Model file for the job. Use its own axes, mm. A direction names the side the tool comes from. Round coordinates to 2 decimals unless told otherwise and drop trailing zeros. Loops run counter-clockwise (first coordinate to the right, second up) from the corner with the lowest first, then second, coordinate; pieces in that order, holes last. Notation, with made-up numbers: (6.5, -4) - (36.5, -4) arc R24 ccw to (36.5, 30) - close; hole circle Ø3 at (-31.5, -13.75). An arc over 180 degrees is marked (long way). Use one line per item in the form item = value.
from build123d import *

# Parameters (mm, degrees)
ESQUISSE1_W                   = 270
ESQUISSE1_H                   = 213
BOSS_EXTRU_1_DEPTH            = 6
ESQUISSE3_R                   = 9.475
ESQUISSE3_R_2                 = 1.5
ENL_V_MAT_EXTRU_1_DEPTH       = 10
ENL_V_MAT_EXTRU_11_DEPTH      = 173.055950202
ENL_V_MAT_EXTRU_11_DEPTH_BACK = 173.055950202
ESQUISSE6_W                   = 40
ESQUISSE6_H                   = 6
BOSS_EXTRU_2_DEPTH            = 6
ESQUISSE7_W                   = 6
ESQUISSE7_H                   = 30
ESQUISSE7_H_2                 = 27
ENL_V_MAT_EXTRU_12_DEPTH      = 6
ESQUISSE8_W                   = 30
ESQUISSE8_H                   = 6
BOSS_EXTRU_3_DEPTH            = 6
ENL_V_MAT_EXTRU_13_DEPTH      = 176.833017377
ENL_V_MAT_EXTRU_14_DEPTH      = 10
ESQUISSE11_W                  = 6
ESQUISSE11_H                  = 15
ENL_V_MAT_EXTRU_15_DEPTH      = 176.833017377
ESQUISSE12_R                  = 1.65
ESQUISSE12_R_2                = 1.185214878
ESQUISSE12_R_3                = 1.5
ENL_V_MAT_EXTRU_16_DEPTH      = 176.833017377
ENL_V_MAT_EXTRU_17_DEPTH      = 176.833017377
ESQUISSE14_R                  = 4
ENL_V_MAT_EXTRU_18_DEPTH      = 1
ESQUISSE15_R                  = 2.995
ESQUISSE15_R_2                = 2.95
ENL_V_MAT_EXTRU_19_DEPTH      = 3
ESQUISSE16_R                  = 1.5
ENL_V_MAT_EXTRU_20_DEPTH      = 10
ESQUISSE17_W                  = 20
ESQUISSE17_H                  = 6
ENL_V_MAT_EXTRU_22_DEPTH      = 10


with BuildPart() as part:
    # Esquisse1 → Boss.-Extru.1 (new body)
    with BuildSketch(Plane.XY):
        Rectangle(ESQUISSE1_W, ESQUISSE1_H)
    extrude(amount=BOSS_EXTRU_1_DEPTH)

    # Esquisse3 → Enlèv. mat.-Extru.1 (cut)
    with BuildSketch(Plane.XY.offset(6)):
        with Locations((-100, -21.5)):
            Circle(ESQUISSE3_R)
        with Locations((43.489676576, 9.523710062)):
            Circle(ESQUISSE3_R_2)
        with Locations((52.149930614, 4.523710062)):
            Circle(ESQUISSE3_R_2)
        with Locations((35.989676576, -3.466670994)):
            Circle(ESQUISSE3_R_2)
        with Locations((44.649930614, -8.466670994)):
            Circle(ESQUISSE3_R_2)
        with Locations((63.702489497, -19.466670994)):
            Circle(ESQUISSE3_R_2)
        with Locations((72.362743535, -24.466670994)):
            Circle(ESQUISSE3_R_2)
        with Locations((79.862743535, -11.476289938)):
            Circle(ESQUISSE3_R_2)
        with Locations((71.202489497, -6.476289938)):
            Circle(ESQUISSE3_R_2)
    extrude(amount=-ENL_V_MAT_EXTRU_1_DEPTH, mode=Mode.SUBTRACT)

    # Esquisse5 → Enlèv. mat.-Extru.11 (cut, two sides: drawn at the far end of the back side and taken through both)
    with BuildSketch(Plane.XY.offset(6).offset(-ENL_V_MAT_EXTRU_11_DEPTH_BACK)):
        Polygon((135, -36.5), (53.963742643, -43.589753853), (-55, -106.5), (135, -106.5), align=None)
    extrude(amount=ENL_V_MAT_EXTRU_11_DEPTH + ENL_V_MAT_EXTRU_11_DEPTH_BACK, mode=Mode.SUBTRACT)

    # Esquisse6 → Boss.-Extru.2 (add)
    with BuildSketch(Plane(origin=(0, 106.5, 0), x_dir=(1, 0, 0), z_dir=(0, 1, 0))):
        with Locations((-75, -3)):
            Rectangle(ESQUISSE6_W, ESQUISSE6_H)
        with Locations((5, -3)):
            Rectangle(ESQUISSE6_W, ESQUISSE6_H)
        with Locations((85, -3)):
            Rectangle(ESQUISSE6_W, ESQUISSE6_H)
    extrude(amount=BOSS_EXTRU_2_DEPTH)

    # Esquisse7 → Enlèv. mat.-Extru.12 (cut)
    with BuildSketch(Plane(origin=(0, 0, 0), x_dir=(-1, 0, 0), z_dir=(0, 0, -1))):
        with Locations((-132, 91.5)):
            Rectangle(ESQUISSE7_W, ESQUISSE7_H)
        with Locations((-132, 34)):
            Rectangle(ESQUISSE7_W, ESQUISSE7_H_2)
        with Locations((-132, -17)):
            Rectangle(ESQUISSE7_W, ESQUISSE7_H_2)
    extrude(amount=-ENL_V_MAT_EXTRU_12_DEPTH, mode=Mode.SUBTRACT)

    # Esquisse8 → Boss.-Extru.3 (add)
    with BuildSketch(Plane.XZ.offset(106.5)):
        with Locations((-95, 3)):
            Rectangle(ESQUISSE8_W, ESQUISSE8_H)
    extrude(amount=BOSS_EXTRU_3_DEPTH)

    # Esquisse9 → Enlèv. mat.-Extru.13 (cut, through all)
    with BuildSketch(Plane(origin=(0, 0, 0), x_dir=(-1, 0, 0), z_dir=(0, 0, -1))):
        Polygon((-110.25, -38.665344422), (-109.727065544, -32.688176234), (-78.422975963, -35.411286132), (-78.863742643, -41.411286132), align=None)
    extrude(amount=-ENL_V_MAT_EXTRU_13_DEPTH, mode=Mode.SUBTRACT)

    # Esquisse10 → Enlèv. mat.-Extru.14 (cut)
    with BuildSketch(Plane(origin=(0, 0, 0), x_dir=(-1, 0, 0), z_dir=(0, 0, -1))):
        Polygon((-32.03555308, -56.25), (-10.384917986, -68.75), (-7.384917986, -63.553847577), (-29.03555308, -51.053847577), align=None)
        Polygon((11.265717109, -81.25), (32.916352203, -93.75), (35.916352203, -88.553847577), (14.265717109, -76.053847577), align=None)
    extrude(amount=-ENL_V_MAT_EXTRU_14_DEPTH, mode=Mode.SUBTRACT)

    # Esquisse11 → Enlèv. mat.-Extru.15 (cut, through all)
    with BuildSketch(Plane(origin=(0, 0, 0), x_dir=(-1, 0, 0), z_dir=(0, 0, -1))):
        with Locations((72, 52)):
            Rectangle(ESQUISSE11_W, ESQUISSE11_H)
        with Locations((72, 83)):
            Rectangle(ESQUISSE11_W, ESQUISSE11_H)
    extrude(amount=-ENL_V_MAT_EXTRU_15_DEPTH, mode=Mode.SUBTRACT)

    # Esquisse12 → Enlèv. mat.-Extru.16 (cut, through all)
    with BuildSketch(Plane(origin=(0, 0, 0), x_dir=(-1, 0, 0), z_dir=(0, 0, -1))):
        with Locations((5, 42.5)):
            Circle(ESQUISSE12_R)
        with Locations((-15, 32.5)):
            Circle(ESQUISSE12_R)
        with Locations((-35, 22.5)):
            Circle(ESQUISSE12_R)
        with Locations((-55, 12.5)):
            Circle(ESQUISSE12_R)
        with Locations((-75, 2.5)):
            Circle(ESQUISSE12_R)
        with Locations((25, 52.5)):
            Circle(ESQUISSE12_R)
        with Locations((45, 62.5)):
            Circle(ESQUISSE12_R)
        with Locations((93, 102.5)):
            Circle(ESQUISSE12_R_2)
        with Locations((3.675250237, 62.5)):
            Circle(ESQUISSE12_R_3)
        with Locations((-15, 52.5)):
            Circle(ESQUISSE12_R_3)
    extrude(amount=-ENL_V_MAT_EXTRU_16_DEPTH, mode=Mode.SUBTRACT)

    # Esquisse13 → Enlèv. mat.-Extru.17 (cut, through all)
    with BuildSketch(Plane(origin=(0, 0, 0), x_dir=(-1, 0, 0), z_dir=(0, 0, -1))):
        Polygon((-129, 76.5), (-129, 106.5), (-105, 106.5), align=None)
    extrude(amount=-ENL_V_MAT_EXTRU_17_DEPTH, mode=Mode.SUBTRACT)

    # Esquisse14 → Enlèv. mat.-Extru.18 (cut)
    with BuildSketch(Plane(origin=(0, 0, 0), x_dir=(-1, 0, 0), z_dir=(0, 0, -1))):
        with Locations((-75, 2.5)):
            Circle(ESQUISSE14_R)
        with Locations((-55, 12.5)):
            Circle(ESQUISSE14_R)
        with Locations((-35, 22.5)):
            Circle(ESQUISSE14_R)
        with Locations((-15, 32.5)):
            Circle(ESQUISSE14_R)
        with Locations((5, 42.5)):
            Circle(ESQUISSE14_R)
        with Locations((25, 52.5)):
            Circle(ESQUISSE14_R)
        with Locations((45, 62.5)):
            Circle(ESQUISSE14_R)
    extrude(amount=-ENL_V_MAT_EXTRU_18_DEPTH, mode=Mode.SUBTRACT)

    # Esquisse15 → Enlèv. mat.-Extru.19 (cut)
    with BuildSketch(Plane(origin=(0, 0, 0), x_dir=(-1, 0, 0), z_dir=(0, 0, -1))):
        with Locations((-85, 109.5)):
            Circle(ESQUISSE15_R)
        with Locations((-5, 109.5)):
            Circle(ESQUISSE15_R)
        with Locations((75, 109.5)):
            Circle(ESQUISSE15_R)
        with Locations((1.940399562, -72.401923789)):
            Circle(ESQUISSE15_R)
        with Locations((-65.76712105, -39.571035308)):
            Circle(ESQUISSE15_R)
        with Locations((45.241669751, -97.401923789)):
            Circle(ESQUISSE15_R_2)
        with Locations((-132, 9.551106058)):
            Circle(ESQUISSE15_R)
        with Locations((-132, 61.579483335)):
            Circle(ESQUISSE15_R)
        with Locations((-119.950479753, -34.805202901)):
            Circle(ESQUISSE15_R)
    extrude(amount=-ENL_V_MAT_EXTRU_19_DEPTH, mode=Mode.SUBTRACT)

    # Esquisse16 → Enlèv. mat.-Extru.20 (cut)
    with BuildSketch(Plane(origin=(0, 0, 0), x_dir=(-1, 0, 0), z_dir=(0, 0, -1))):
        with Locations((-5, 109.5)):
            Circle(ESQUISSE16_R)
        with Locations((74.967795866, 109.5)):
            Circle(ESQUISSE16_R)
        with Locations((-85, 109.5)):
            Circle(ESQUISSE16_R)
        with Locations((-132, 61.579483335)):
            Circle(ESQUISSE16_R)
        with Locations((-132, 9.551106058)):
            Circle(ESQUISSE16_R)
        with Locations((-119.950479753, -34.805202901)):
            Circle(ESQUISSE16_R)
        with Locations((-65.76712105, -39.571035308)):
            Circle(ESQUISSE16_R)
        with Locations((1.940399562, -72.401923789)):
            Circle(ESQUISSE16_R)
        with Locations((45.241669751, -97.401923789)):
            Circle(ESQUISSE16_R)
    extrude(amount=-ENL_V_MAT_EXTRU_20_DEPTH, mode=Mode.SUBTRACT)

    # Esquisse17 → Enlèv. mat.-Extru.22 (cut)
    with BuildSketch(Plane(origin=(0, 0, 0), x_dir=(-1, 0, 0), z_dir=(0, 0, -1))):
        with Locations((105, 53)):
            Rectangle(ESQUISSE17_W, ESQUISSE17_H)
    extrude(amount=-ENL_V_MAT_EXTRU_22_DEPTH, mode=Mode.SUBTRACT)


solid = part.part
1. Wall check: probe 1 along Y at (x, z) = (-45, 0.85); probe 2 along Y at (x, z) = (-104.5, 3.75); probe 3 along X at (y, z) = (53, 4.25). Give the ranges that are in metal, low to high.
Geometry check:
probe_1 = -100.73 to -100.34, -94.46 to 58.5, 66.5 to 106.5
probe_2 = -112.5 to -29.84, -13.16 to 50, 56 to 106.5
probe_3 = -135 to -115, -95 to -75, -69 to -26.57, -23.43 to 13.59, 16.41 to 135
2. Cut at A-A, the plane x = -100. Give the cut face in (y, z) (3 decimals), plus the area to 3 significant figures.
Geometry check:
outline = (-112.5, 0) - (-30.975, 0) - (-30.975, 6) - (-112.5, 6) - close; (-12.025, 0) - (50, 0) - (50, 6) - (-12.025, 6) - close; (56, 0) - (106.5, 0) - (106.5, 6) - (56, 6) - close
area = 1,160 mm^2
3. Tool access for faces 4 (the flat face through (-35, 106.5, 3)), 5 (the flat face through (-115, 53, 3)), 6 (the flat face through (129, 34, 3)), 7 (the cylindrical face through (5.649, 106.576, 1.479)): list every direction of +Z, -Z, +X, -X, +Y, -Y with a clear straight run to the whole face (end or side of a thin tool).
Geometry check:
face_4 = +Z, -Z, +Y
face_5 = +Z, -Z
face_6 = +Z, -Z, +X
face_7 = -Z
4. Pull direction Y, two halves, no side cores. Call faces 1 (the flat face through (45, 106.5, 3)), 2 (the cylindrical face through (-46.6, -100.02, 1.48)), 3 (the flat face through (-110, -109, 3)): +Y half, -Y half, draft (parallel to the pull), parting line (faces both ways), or undercut.
Geometry check:
face_1 = +Y half
face_2 = undercut
face_3 = draft
5. Flat gauge pins, fed straight in: pin 1 (4 mm diameter, centred on x = 35.99, y = -3.47, fed in from +Z); pin 2 (4 mm diameter, centred on x = -23.5, y = 51.5, fed in from -Z); pin 3 (3.5 mm diameter, centred on x = 132, y = 9.55, fed in from -Z); pin 4 (3 mm diameter, centred on x = 53, z = 1, fed in from +Y). Where does each tip first touch, or does it go through?
Geometry check:
pin_1 = 6
pin_2 = 1
pin_3 = 3
pin_4 = 106.5
6. Cut at B-B, the plane z = 4.25. Give the number of separate pieces and of enclosed holes in the cut face, plus the area to 3 significant figures.
Geometry check:
separate_pieces = 1
enclosed_holes = 31
area = 47,500 mm^2
